Verification items for the finished model (mm, model axes). Give positions to 0.01 mm unless a question says otherwise; leave off trailing zeros. Write each loop counter-clockwise with the first axis right and the second up, starting at its lowest first coordinate (ties: lowest second). Pieces come first, ordered by that corner, then holes. Notation, with made-up numbers: (32, -30.75) - (89, -30.75) arc R13 ccw to (89, -5.75) - close; hole circle Ø7 at (74, 7). An arc over 180 degrees is marked (long way). Answer as a JSON object with one key per item and string values. Group by question number.
Item 1: Sectioned sample at D-D, the plane x = 0.5. Record the boundary of the cut face in (y, z), and give its area (3 significant figures).
Item 2: Scan lines: line 1 along X through (y, z) = (-132, 0.25); line 2 along Z through (x, y) = (-1, -25). Record each from-to range of solid material in increasing order. Write a range as [from, to].
Item 3: Sectioned sample at A-A, the plane y = -8. Record the boundary of the cut face in (x, z), and give its area (3 significant figures).
Item 4: Sectioned sample at B-B, the plane y = -80. Record the boundary of the cut face in (x, z).
Item 5: Go/stop test with flat-tipped pins: pin 1 (4.5 mm diameter, centred on y = -104, z = 0, fed in from -X); pin 2 (2 mm diameter, centred on x = 0, y = -39.5, fed in from +Z). Record where each tip stops, or that it passes through.
Item 6: Sectioned sample at C-C, the plane z = 0. Count the separate pieces of the cut face and the enclosed holes in it, and give its area (4 significant figures).
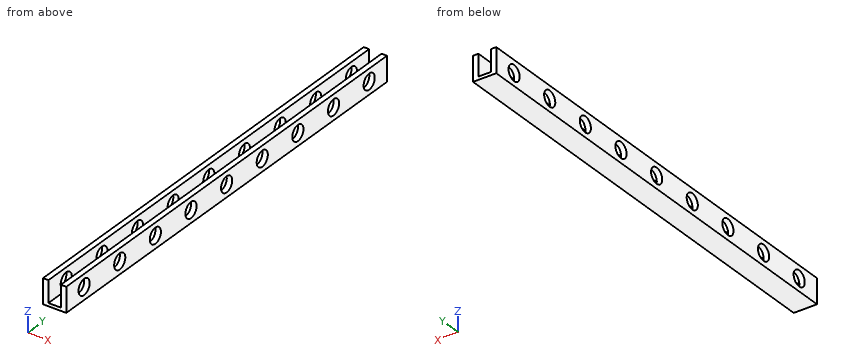
```python
from build123d import *

# Parameters (mm, degrees)
BASE_DEPTH  = 144
ESQUISSE2_R = 2.5
TROU_DEPTH  = 145.250649912


with BuildPart() as part:
    # Esquisse1 → Base (new body)
    with BuildSketch(Plane(origin=(0, 0, 0), x_dir=(1, 0, 0), z_dir=(0, 1, 0))):
        Polygon((-2, -4), (-2, 3), (2, 3), (2, -4), (3.75, -4), (3.75, 4), (-3.75, 4), (-3.75, -4), align=None)
    extrude(amount=-BASE_DEPTH)

    # Esquisse2 → Trou (cut, through all)
    with BuildSketch(Plane.ZY.offset(3.75)):
        with Locations((0, -8)):
            Circle(ESQUISSE2_R)
        with Locations((0, -24)):
            Circle(ESQUISSE2_R)
        with Locations((0, -40)):
            Circle(ESQUISSE2_R)
        with Locations((0, -56)):
            Circle(ESQUISSE2_R)
        with Locations((0, -72)):
            Circle(ESQUISSE2_R)
        with Locations((0, -88)):
            Circle(ESQUISSE2_R)
        with Locations((0, -104)):
            Circle(ESQUISSE2_R)
        with Locations((0, -120)):
            Circle(ESQUISSE2_R)
        with Locations((0, -136)):
            Circle(ESQUISSE2_R)
    extrude(amount=-TROU_DEPTH, mode=Mode.SUBTRACT)


solid = part.part
```
Geometry check:
{
 "1": {"outline": "(-144, -4) - (0, -4) - (0, -3) - (-144, -3) - close", "area": "144 mm^2"},
 "2": {"line 1": "[-3.75, -2], [2, 3.75]", "line 2": "[-4, -3]"},
 "3": {"outline": "(-3.75, -4) - (3.75, -4) - (3.75, -2.5) - (2, -2.5) - (2, -3) - (-2, -3) - (-2, -2.5) - (-3.75, -2.5) - close; (-3.75, 2.5) - (-2, 2.5) - (-2, 4) - (-3.75, 4) - close; (2, 2.5) - (3.75, 2.5) - (3.75, 4) - (2, 4) - close", "area": "14.5 mm^2"},
 "4": {"outline": "(-3.75, -4) - (3.75, -4) - (3.75, 4) - (2, 4) - (2, -3) - (-2, -3) - (-2, 4) - (-3.75, 4) - close"},
 "5": {"pin 1": "through", "pin 2": "z = -3"},
 "6": {"separate pieces": "20", "enclosed holes": "0", "area": "346.5 mm^2"}
}
